```python
from build123d import *

# Parameters (mm, degrees)
SKETCH1_W           = 50
SKETCH1_H           = 20
SKETCH1_R           = 1.75
BOSS_EXTRUDE1_DEPTH = 1.6
SKETCH3_R           = 0.35
CUT_EXTRUDE1_DEPTH  = 2.6


with BuildPart() as part:
    # Sketch1 → Boss-Extrude1 (new body)
    with BuildSketch(Plane(origin=(0, 0, 0), x_dir=(1, 0, 0), z_dir=(0, 1, 0))):
        with Locations((25, 10)):
            Rectangle(SKETCH1_W, SKETCH1_H)
        with Locations((3, 17)):
            Circle(SKETCH1_R, mode=Mode.SUBTRACT)
        with Locations((47, 3)):
            Circle(SKETCH1_R, mode=Mode.SUBTRACT)
        with Locations((3, 3)):
            Circle(SKETCH1_R, mode=Mode.SUBTRACT)
        with Locations((47, 17)):
            Circle(SKETCH1_R, mode=Mode.SUBTRACT)
    extrude(amount=BOSS_EXTRUDE1_DEPTH)

    # Sketch3 → Cut-Extrude1 (cut, through all)
    with BuildSketch(Plane(origin=(0, 1.6, 0), x_dir=(1, 0, 0), z_dir=(0, 1, 0))):
        with Locations((9.25, 0.75)):
            Circle(SKETCH3_R)
        with Locations((10.75, 0.75)):
            Circle(SKETCH3_R)
        with Locations((10.75, 5.5)):
            Circle(SKETCH3_R)
        with Locations((10.75, 14.5)):
            Circle(SKETCH3_R)
        with Locations((15.75, 5.5)):
            Circle(SKETCH3_R)
        with Locations((15.75, 14.5)):
            Circle(SKETCH3_R)
        with Locations((15.75, 0.75)):
            Circle(SKETCH3_R)
        with Locations((14.25, 0.75)):
            Circle(SKETCH3_R)
        with Locations((20.75, 5.5)):
            Circle(SKETCH3_R)
        with Locations((20.75, 14.5)):
            Circle(SKETCH3_R)
        with Locations((20.75, 0.75)):
            Circle(SKETCH3_R)
        with Locations((19.25, 0.75)):
            Circle(SKETCH3_R)
        with Locations((25.75, 5.5)):
            Circle(SKETCH3_R)
        with Locations((25.75, 14.5)):
            Circle(SKETCH3_R)
        with Locations((25.75, 0.75)):
            Circle(SKETCH3_R)
        with Locations((24.25, 0.75)):
            Circle(SKETCH3_R)
        with Locations((30.75, 5.5)):
            Circle(SKETCH3_R)
        with Locations((30.75, 14.5)):
            Circle(SKETCH3_R)
        with Locations((30.75, 0.75)):
            Circle(SKETCH3_R)
        with Locations((29.25, 0.75)):
            Circle(SKETCH3_R)
        with Locations((35.75, 5.5)):
            Circle(SKETCH3_R)
        with Locations((35.75, 14.5)):
            Circle(SKETCH3_R)
        with Locations((35.75, 0.75)):
            Circle(SKETCH3_R)
        with Locations((34.25, 0.75)):
            Circle(SKETCH3_R)
        with Locations((40.75, 5.5)):
            Circle(SKETCH3_R)
        with Locations((40.75, 14.5)):
            Circle(SKETCH3_R)
        with Locations((40.75, 0.75)):
            Circle(SKETCH3_R)
        with Locations((39.25, 0.75)):
            Circle(SKETCH3_R)
    extrude(amount=-CUT_EXTRUDE1_DEPTH, mode=Mode.SUBTRACT)


solid = part.part
```
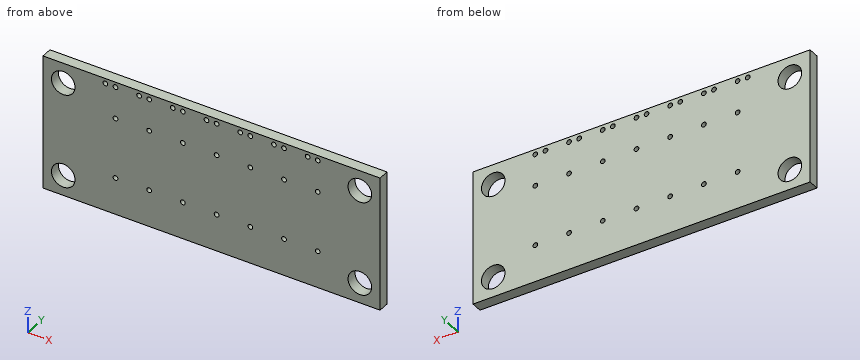
CAD build for the part. Positions are in the model's coordinates, mm. Coordinates: 2 decimals unless noted, no trailing zeros. Loops run counter-clockwise (first coordinate to the right, second up) from the corner with the lowest first, then second, coordinate; pieces in that order, holes last. Notation, with made-up numbers: (-32, 72) - (-15, 72) arc R22 cw to (-15, 111) - close; hole circle Ø5 at (68.25, -31). An arc over 180 degrees is marked (long way). Return JSON: item names as keys, results as strings.
1. Band-saw the part on C-C (y = 0.8). State how many separate pieces and enclosed holes the cut face has, and give its area (3 significant figures).
Result:
{"separate pieces": "1", "enclosed holes": "32", "area": "951 mm2"}
2. Probe L1, parallel to Z at x = 20.75, y = 0.4; L2, parallel to X at y = 0.9, z = -17; L3, parallel to X at y = 0.25, z = -3.75. List the from-to ranges inside material, lowest first. Write a range as from..to.
Result:
{"L1": "z = -20..-14.85, -14.15..-5.85, -5.15..-1.1, -0.4..0", "L2": "x = 0..1.25, 4.75..45.25, 48.75..50", "L3": "x = 0..1.42, 4.58..45.42, 48.58..50"}
3. Band-saw the part on A-A (z = -3.5). Give the cut face in (x, y).
Result:
{"outline": "(0, 0) - (1.32, 0) - (1.32, 1.6) - (0, 1.6) - close; (4.68, 0) - (45.32, 0) - (45.32, 1.6) - (4.68, 1.6) - close; (48.68, 0) - (50, 0) - (50, 1.6) - (48.68, 1.6) - close"}
4. Band-saw the part on B-B (z = -16). Give the cut face in (x, y), and give its area (3 significant figures).
Result:
{"outline": "(0, 0) - (1.56, 0) - (1.56, 1.6) - (0, 1.6) - close; (4.44, 0) - (45.56, 0) - (45.56, 1.6) - (4.44, 1.6) - close; (48.44, 0) - (50, 0) - (50, 1.6) - (48.44, 1.6) - close", "area": "70.8 mm2"}
